Input: part model. Units: mm. Frame: model coordinates. A direction names the side the tool comes from. Give positions to 0.01 mm unless a question says otherwise; leave off trailing zeros. Write each loop counter-clockwise with the first axis right and the second up, starting at its lowest first coordinate (ties: lowest second). Pieces come first, ordered by that corner, then holes. Notation, with made-up numbers: (76, 42.5) -> (106, 42.5) arc R27 cw to (106, 70.5) -> close; hole circle Ø9 at (67, -39.5). An arc over 180 degrees is marked (long way). Return JSON: item names as keys, results as strings. Group by question number.
Item 1: Section B-B, the plane z = -23. Return loops of the section in (x, y).
Item 2: Mould query, pull axis Z, two halves, no side actions, for faces 1 (the face through (15, 13, -68.58)), 2 (the face through (19, 3.81, -4)), 3 (the face through (20, 3, -7.62)). Classes: released by +Z, released by -Z, zero draft, split by the parting line, or undercut.
Item 3: Section A-A, the plane z = -37. Return loops of the section in (x, y), then the cut area to 3 significant figures.
Item 4: Pin query (flat end, axial travel): P1, Ø1.5, axis at x = 10, y = 18, coming from the +Z side; P2, Ø2.5, axis at x = 21.5, y = 12, coming from the -Z side; P3, Ø4, axis at x = 29, z = -74, coming from the +Y side. Return the tip coordinate at first contact, or that it passes through.
Item 5: Section D-D, the plane y = 15.5. Return loops of the section in (x, z), then the cut area to 3 significant figures.
Item 6: Set-up query: faces 4 (the face through (31, 3, -68.58)), 5 (the face through (10, 1, -17.78)), 6 (the face through (3, 3, -68.58)). Return all of +Z, -Z, +X, -X, +Y, -Y with unobstructed straight access to the full face (end or side cutting, diameter ignored); none if empty.
Item 7: Line query: line 1 (Z direction, x = 17, y = 2.5); line 2 (X direction, y = 2.25, z = -16); line 3 (Z direction, x = 9, y = 18.25). Output: solid intervals per line, ascending. Write a range as [from, to].
Item 8: Section C-C, the plane y = 12. Return loops of the section in (x, z), then the cut area to 3 significant figures.
from build123d import *

# Parameters (mm, degrees)
BOSS_EXTRUDE2_DEPTH   = 3.81
BOSS_EXTRUDE2_2_DEPTH = 3.81
SKETCH2_3_W           = 39.3827
SKETCH2_3_H           = 60.96
SKETCH2_3_R           = 2.794
SKETCH2_3_W_2         = 7.874
SKETCH2_3_H_2         = 50.8
BOSS_EXTRUDE3_DEPTH   = 2.286
SKETCH2_4_W           = 0.75
SKETCH2_4_H           = 50.8
BOSS_EXTRUDE4_DEPTH   = 22.86
SKETCH4_W             = 50.8
SKETCH4_H             = 0.889
BOSS_EXTRUDE5_DEPTH   = 12.7
BOSS_EXTRUDE7_DEPTH   = 0.762
BOSS_EXTRUDE8_DEPTH   = 50.8
BOSS_EXTRUDE11_START  = 46.99
BOSS_EXTRUDE11_DEPTH  = 3.81
SKETCH8_W             = 10.208213857
SKETCH8_H             = 50.038
CUT_EXTRUDE2_DEPTH    = 89.208426668


# Read off the part's stored shape, not the designer's step: Boss-Extrude8
with BuildPart() as part:
    # Sketch2 → Boss-Extrude2 (new body)
    with BuildSketch(Plane(origin=(0, 0, 0), x_dir=(1, 0, 0), z_dir=(0, 1, 0))):
        Polygon((0, 7.62), (0, 0), (39.3827, 0), (39.3827, 7.62), (7.62, 7.62), (6.87, 7.62), align=None)
    extrude(amount=BOSS_EXTRUDE2_DEPTH)



with BuildPart() as body_2:
    # Sketch2 → Boss-Extrude2 2 (new body)
    with BuildSketch(Plane(origin=(0, 0, 0), x_dir=(1, 0, 0), z_dir=(0, 1, 0))):
        Polygon((0, 76.2), (0, 68.58), (6.87, 68.58), (7.62, 68.58), (39.3827, 68.58), (39.3827, 76.2), align=None)
    extrude(amount=BOSS_EXTRUDE2_2_DEPTH)


with BuildPart() as part_1:
    add(part.part)

    add(body_2.part)  # Boss-Extrude3 merges body 2
    # Sketch2<3> → Boss-Extrude3 (add)
    with BuildSketch(Plane(origin=(0, 0, 0), x_dir=(1, 0, 0), z_dir=(0, 1, 0))):
        with Locations((19.69135, 38.1)):
            Rectangle(SKETCH2_3_W, SKETCH2_3_H)
        with Locations(Location((30.067932262, 53.467, 0), (0, 0, 270))):
            Circle(SKETCH2_3_R, mode=Mode.SUBTRACT)
        with Locations((15.113, 38.1)):
            Rectangle(SKETCH2_3_W_2, SKETCH2_3_H_2, mode=Mode.SUBTRACT)
        with Locations(Location((30.067932262, 22.733, 0), (0, 0, 270))):
            Circle(SKETCH2_3_R, mode=Mode.SUBTRACT)
    extrude(amount=BOSS_EXTRUDE3_DEPTH)

    # Sketch2<4> → Boss-Extrude4 (add)
    with BuildSketch(Plane(origin=(0, 0, 0), x_dir=(1, 0, 0), z_dir=(0, 1, 0))):
        with Locations((7.245, 43.18)):
            Rectangle(SKETCH2_4_W, SKETCH2_4_H)
    extrude(amount=BOSS_EXTRUDE4_DEPTH)

    # Sketch4 → Boss-Extrude5 (add)
    with BuildSketch(Plane(origin=(7.62, 0, 0), x_dir=(0, 0, -1), z_dir=(1, 0, 0))):
        with Locations((43.18, 22.4155)):
            Rectangle(SKETCH4_W, SKETCH4_H)
    extrude(amount=BOSS_EXTRUDE5_DEPTH)

    # Sketch6 → Boss-Extrude7 (add)
    with BuildSketch(Plane.XY.offset(-68.58)):
        Polygon((7.62, 2.286), (23.50135, 2.286), (23.255051935, 3.81), (22.483164843, 3.81), (19.548112907, 21.971), (7.62, 21.971), align=None)
    extrude(amount=BOSS_EXTRUDE7_DEPTH)

    # Boss-Extrude8 outline → Boss-Extrude8 (add)
    with BuildSketch(Plane.XY.offset(-68.58)):
        Polygon((20.32, 21.971), (17.64673175, 21.971), (19.826070786, 20.25110095), (22.532645041, 3.503835102), (19.548112907, 2.286), (23.50135, 2.286), align=None)
        Polygon((7.62, 20.25110095), (9.33989905, 21.971), (7.62, 21.971), align=None)
        Polygon((7.62, 2.286), (9.33989905, 2.286), (7.62, 2.98989905), align=None)
    extrude(amount=BOSS_EXTRUDE8_DEPTH)

    # Sketch6<6> → Boss-Extrude11 (add)
    with BuildSketch(Plane.XY.offset(-68.58).offset(BOSS_EXTRUDE11_START)):
        Polygon((19.548112907, 20.470460804), (19.548112907, 2.286), (22.532645041, 3.503835102), (19.826070786, 20.25110095), align=None)
    extrude(amount=BOSS_EXTRUDE11_DEPTH)

    # Sketch8 → Cut-Extrude2 (cut, through all)
    with BuildSketch(Plane(origin=(0, 2.286, 0), x_dir=(1, 0, 0), z_dir=(0, 1, 0))):
        with Locations((14.444005979, 42.799)):
            Rectangle(SKETCH8_W, SKETCH8_H)
    extrude(amount=-CUT_EXTRUDE2_DEPTH, mode=Mode.SUBTRACT)


solid = part_1.part
Answer below:
{
 "1": {"outline": "(0, 0) -> (9.34, 0) -> (9.34, 2.29) -> (7.62, 2.99) -> (7.62, 20.25) -> (9.34, 21.97) -> (17.65, 21.97) -> (19.83, 20.25) -> (22.53, 3.5) -> (19.55, 2.29) -> (19.55, 0) -> (27.29, 0) -> (27.29, 2.29) -> (23.5, 2.29) -> (20.32, 21.97) -> (20.32, 22.86) -> (6.87, 22.86) -> (6.87, 2.29) -> (0, 2.29) -> close; (32.85, 0) -> (39.38, 0) -> (39.38, 2.29) -> (32.85, 2.29) -> close"},
 "2": {"face 1": "released by -Z", "face 2": "zero draft", "face 3": "undercut"},
 "3": {"outline": "(0, 0) -> (9.34, 0) -> (9.34, 2.29) -> (7.62, 2.99) -> (7.62, 20.25) -> (9.34, 21.97) -> (17.65, 21.97) -> (19.83, 20.25) -> (22.53, 3.5) -> (19.55, 2.29) -> (19.55, 0) -> (39.38, 0) -> (39.38, 2.29) -> (23.5, 2.29) -> (20.32, 21.97) -> (20.32, 22.86) -> (6.87, 22.86) -> (6.87, 2.29) -> (0, 2.29) -> close", "area": "114 mm2"},
 "4": {"P1": "stops at z = -67.82", "P2": "stops at z = -68.58", "P3": "stops at y = 3.81"},
 "5": {"outline": "(6.87, -68.58) -> (21.37, -68.58) -> (21.37, -17.78) -> (19.55, -17.78) -> (19.55, -21.59) -> (20.59, -21.59) -> (20.59, -67.82) -> (7.62, -67.82) -> (7.62, -17.78) -> (6.87, -17.78) -> close", "area": "91.2 mm2"},
 "6": {"face 4": "+X, +Y", "face 5": "-Y", "face 6": "-X, +Y"},
 "7": {"line 1": "z = [-76.2, -67.82], [-7.62, 0]", "line 2": "x = [0, 11.18], [19.05, 39.38]", "line 3": "z = [-68.58, -67.82]"},
 "8": {"outline": "(6.87, -68.58) -> (21.93, -68.58) -> (21.93, -17.78) -> (19.55, -17.78) -> (19.55, -21.59) -> (21.16, -21.59) -> (21.16, -67.82) -> (7.62, -67.82) -> (7.62, -17.78) -> (6.87, -17.78) -> close", "area": "93.8 mm2"}
}
